```python
from build123d import *

# Parameters (mm, degrees)
F0_W        = 228.6
F0_H        = 76.2
F1_DEPTH    = 457.2
F2_SIZE     = 25.4
F3_W        = 59.69
F3_H        = 360
F4_DEPTH    = 76.2
F1_FACE_W   = 177.8
F1_FACE_H   = 457.2
F1_FACE_W_2 = 119.38
F1_FACE_H_2 = 360
F5_DEPTH    = 6.35
F6_DEPTH    = 31.75


with BuildPart() as f1:
    # F0 (on Top) → F1 (new body)
    with BuildSketch(Plane.XY):
        Rectangle(F0_W, F0_H)
    extrude(amount=F1_DEPTH)

    # F2
    f2_edges = [f1.edges().sort_by_distance(p)[0] for p in [
        (-114.3, -38.1, 228.6),
        (114.3, -38.1, 228.6),
    ]]
    chamfer(f2_edges, length=F2_SIZE)

    # F3 (on face) → F4 (cut)
    with BuildSketch(Plane.XZ.offset(38.1)):
        with Locations((29.845, 235.544)):
            Rectangle(F3_W, F3_H)
        with Locations((-29.845, 235.544)):
            Rectangle(F3_W, F3_H)
    extrude(amount=-F4_DEPTH, mode=Mode.SUBTRACT)

    # F3 (on face) + F1_face (on face) → F5 (cut)
    with BuildSketch(Plane.XZ.offset(38.1)):
        Polygon((-76.2, 12.7), (0, 12.7), (0, 55.544), (-59.69, 55.544), (-59.69, 415.544), (0, 415.544), (0, 444.5), (-76.2, 444.5), align=None)
        Polygon((0, 55.544), (0, 12.7), (76.2, 12.7), (76.2, 444.5), (0, 444.5), (0, 415.544), (59.69, 415.544), (59.69, 55.544), align=None)
    with BuildSketch(Plane(origin=(0, -38.1, 228.6), x_dir=(1, 0, 0), z_dir=(0, -1, 0))):
        Rectangle(F1_FACE_W, F1_FACE_H)
        with Locations((0, 6.944)):
            Rectangle(F1_FACE_W_2, F1_FACE_H_2, mode=Mode.SUBTRACT)
    extrude(amount=-F5_DEPTH, mode=Mode.SUBTRACT)

    # F3 (on face) → F6 (cut)
    with BuildSketch(Plane.XZ.offset(38.1)):
        Polygon((0, 55.544), (0, 12.7), (76.2, 12.7), (76.2, 444.5), (0, 444.5), (0, 415.544), (59.69, 415.544), (59.69, 55.544), align=None)
        Polygon((-76.2, 12.7), (0, 12.7), (0, 55.544), (-59.69, 55.544), (-59.69, 415.544), (0, 415.544), (0, 444.5), (-76.2, 444.5), align=None)
    extrude(amount=-F6_DEPTH, mode=Mode.SUBTRACT)


solid = f1.part
```
Geometry check sheet. Reference: the model listing, model coordinates, mm. A direction names the side the tool comes from. Coordinates: 2 decimals unless noted, no trailing zeros. Loops run counter-clockwise (first coordinate to the right, second up) from the corner with the lowest first, then second, coordinate; pieces in that order, holes last. Notation, with made-up numbers: (5.5, -23) -> (11.5, -23) arc R20 cw to (11.5, 6) -> close; hole circle Ø6 at (18, 31). An arc over 180 degrees is marked (long way). Put each result on its own line as item: value.
1) Cross-section at C-C on z = 193. Record the boundary of the cut face in (x, y), plus the area to 3 significant figures.
Result set:
outline: (-114.3, -12.7) -> (-88.9, -38.1) -> (-88.9, -31.75) -> (-76.2, -31.75) -> (-76.2, -6.35) -> (-59.69, -6.35) -> (-59.69, 38.1) -> (-114.3, 38.1) -> close; (59.69, -6.35) -> (76.2, -6.35) -> (76.2, -31.75) -> (88.9, -31.75) -> (88.9, -38.1) -> (114.3, -12.7) -> (114.3, 38.1) -> (59.69, 38.1) -> close
area: 6,470 mm^2
2) Cross-section at D-D on z = 45. Record the boundary of the cut face in (x, y).
Result set:
outline: (-114.3, -12.7) -> (-88.9, -38.1) -> (-88.9, -31.75) -> (-76.2, -31.75) -> (-76.2, -6.35) -> (76.2, -6.35) -> (76.2, -31.75) -> (88.9, -31.75) -> (88.9, -38.1) -> (114.3, -12.7) -> (114.3, 38.1) -> (-114.3, 38.1) -> close
3) Cross-section at A-A on y = 17.5. Record the boundary of the cut face in (x, z).
Result set:
outline: (-114.3, 0) -> (114.3, 0) -> (114.3, 457.2) -> (-114.3, 457.2) -> close; hole (-59.69, 55.54) -> (59.69, 55.54) -> (59.69, 415.54) -> (-59.69, 415.54) -> close
4) Thickness scan on line 1 (X direction, y = 29.5, z = 414.5); line 2 (Z direction, x = -58, y = 6.5); line 3 (Z direction, x = 59.5, y = -14.5). Record the ranges inside material, lowest first.
Result set:
line 1: x = -114.3 to -59.69, 59.69 to 114.3
line 2: z = 0 to 55.54, 415.54 to 457.2
line 3: z = 0 to 12.7, 444.5 to 457.2
5) Cross-section at B-B on x = 39.5. Record the boundary of the cut face in (y, z).
Result set:
outline: (-31.75, 0) -> (38.1, 0) -> (38.1, 55.54) -> (-6.35, 55.54) -> (-6.35, 12.7) -> (-31.75, 12.7) -> close; (-31.75, 444.5) -> (-6.35, 444.5) -> (-6.35, 415.54) -> (38.1, 415.54) -> (38.1, 457.2) -> (-31.75, 457.2) -> close
6) Gauge pin test, flat ends, axial feed: pin 1 Ø1.9 at (y, z) = (-35.5, 244.5) entering from -X; pin 2 Ø8 at (y, z) = (-19, 347) entering from +X; pin 3 Ø3 at (x, z) = (-18.5, 48.5) entering from -Y. Record the tip position at first contact, or that the pin passes through.
Result set:
pin 1: stops at x = -92.45
pin 2: stops at x = 112
pin 3: stops at y = -6.35
7) Tool access check on faces 1 (the flat face through (-1, -19, 12.7)), 2 (the flat face through (-79, -31.75, 247)), 3 (the flat face through (114.3, 12, 225)), 4 (the flat face through (-59.69, 16, 233)). Record the directions out of +Z, -Z, +X, -X, +Y, -Y that give a thin tool (end or side, any length) a straight path to the whole face; none if there is none.
Result set:
face 1: -Y
face 2: +Z, -Z, -Y
face 3: +Z, -Z, +X, +Y, -Y
face 4: +Y, -Y
8) Release check for a two-part mould opening along Z. For faces 5 (the flat face through (-78, 38.1, 225)), 6 (the flat face through (-2, 9, 0)), 7 (the flat face through (59.69, 16, 233)) record: released by +Z, released by -Z, zero draft, split by the parting line, or undercut.
Result set:
face 5: zero draft
face 6: released by -Z
face 7: undercut
